from build123d import *

# Parameters (mm, degrees)
F0_R          = 38.3309835302
F0_R_2        = 24.0387523189
F1_DEPTH      = 101.6
F2_W          = 25.4
F2_H          = 50.8
F3_DEPTH      = 38.3319835302
F3_DEPTH_BACK = 38.3319835302
F4_R          = 4.4552500981
F5_DEPTH      = 25.4


with BuildPart() as f1:
    # F0 (on Top) → F1 (new body)
    with BuildSketch(Plane.XY):
        Circle(F0_R)
        Circle(F0_R_2, mode=Mode.SUBTRACT)
    extrude(amount=F1_DEPTH)

    # F2 (on Front) → F3 (cut, two sides)
    with BuildSketch(Plane.XZ) as f3_sk:
        with Locations((0, 50.8)):
            Rectangle(F2_W, F2_H)
    extrude(amount=-F3_DEPTH, mode=Mode.SUBTRACT)
    extrude(f3_sk.sketch, amount=F3_DEPTH_BACK, mode=Mode.SUBTRACT)

    # F4 (on face) → F5 (cut, through all)
    with BuildSketch(Plane.XY.offset(101.6)):
        with Locations((0, 31.9115035236)):
            Circle(F4_R)
    extrude(amount=-F5_DEPTH, mode=Mode.SUBTRACT)


solid = f1.part
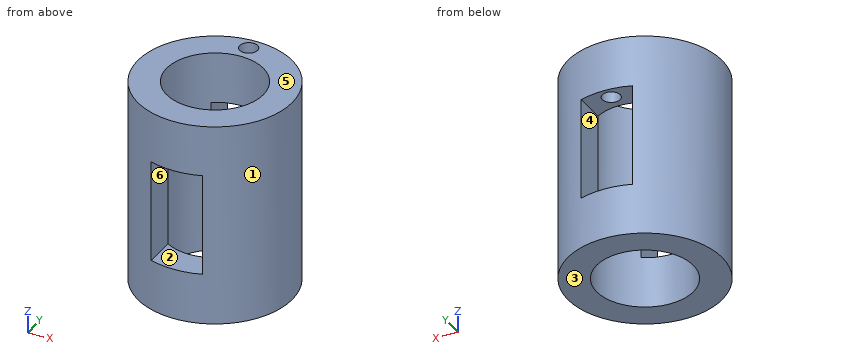
Could you check a few things on this model? Use its own coordinates, in mm. Face numbers are marked on the shaded views. A direction names the side the tool comes from. Give positions to 0.01 mm unless a question says otherwise; leave off trailing zeros. Loops run counter-clockwise (first coordinate to the right, second up) from the corner with the lowest first, then second, coordinate; pieces in that order, holes last. Notation, with made-up numbers: M -39.5,-6 L -35.5,-6 A14 cw -35.5,-1 Z; hole C 5,65.25 d9. An arc over 180 degrees is marked long. Answer as a JSON object with one key per item and string values.
Q1. For P1, Ø6, axis at y = 17, z = 21.5, coming from the +X side; P2, Ø6, axis at x = -27, z = 74, coming from the +Y side; P3, Ø4.5, axis at y = 31.5, z = 52.5, coming from the -X side, each with a flat end and sliding along its axis, tell me the tip position at first contact or that it passes through.
Values found:
{"P1": "stops at x = 35.68", "P2": "stops at y = 29.89", "P3": "stops at x = -24.77"}
Q2. If I drill on probe 1 along Y at (x, z) = (0, 80.5); probe 2 along X at (y, z) = (-0.5, 65.5); probe 3 along X at (y, z) = (-12, 79), over which ranges is the centre line in solid material (lowest first)? Write a range as [from, to].
Values found:
{"probe 1": "y = [-38.33, -24.04], [24.04, 27.46], [36.37, 38.33]", "probe 2": "x = [-38.33, -24.03], [24.03, 38.33]", "probe 3": "x = [-36.4, -20.83], [20.83, 36.4]"}
Q3. Suppose I cut it at D-D, the plane x = -9. List the corners of the cut face in (y, z) for me.
Values found:
{"outline": "M -37.26,0 L -22.29,0 L -22.29,25.4 L -37.26,25.4 Z; M -37.26,76.2 L -22.29,76.2 L -22.29,101.6 L -37.26,101.6 Z; M 22.29,0 L 37.26,0 L 37.26,25.4 L 22.29,25.4 Z; M 22.29,76.2 L 37.26,76.2 L 37.26,101.6 L 22.29,101.6 Z"}
Q4. If we mould it in two halves opening along X, with no side actions, what happens to the marked faces 1, 2, 3 and 4? For each: pulls with the +X half, pulls with the -X half, needs draft (parallel to the pull), parting line crosses it, or undercut.
Values found:
{"face 1": "parting line crosses it", "face 2": "undercut", "face 3": "needs draft", "face 4": "undercut"}
Q5. Suppose I cut it at C-C, the plane z = 53. List the corners of the cut face in (x, y) for me, plus the area to 3 significant figures.
Values found:
{"outline": "M -12.7,-36.17 L -12.7,-20.41 A24.04 cw -12.7,20.41 L -12.7,36.17 A38.33 ccw Z; M 12.7,-36.17 A38.33 ccw 12.7,36.17 L 12.7,20.41 A24.04 cw 12.7,-20.41 Z", "area": "2,050 mm²"}
Q6. For the marked faces 5 and 6, which set-ups out of +Z, -Z, +X, -X, +Y, -Y let a thin tool reach every point of the face, with its end or its side?
Values found:
{"face 5": "+Z, +X, -X, +Y, -Y", "face 6": "+Y, -Y"}
Q7. Suppose I cut it at B-B, the plane x = 0. List the corners of the cut face in (y, z) for me.
Values found:
{"outline": "M -38.33,0 L -24.04,0 L -24.04,25.4 L -38.33,25.4 Z; M -38.33,76.2 L -24.04,76.2 L -24.04,101.6 L -38.33,101.6 Z; M 24.04,0 L 38.33,0 L 38.33,25.4 L 24.04,25.4 Z; M 24.04,76.2 L 27.46,76.2 L 27.46,101.6 L 24.04,101.6 Z; M 36.37,76.2 L 38.33,76.2 L 38.33,101.6 L 36.37,101.6 Z"}
Q8. Suppose I cut it at A-A, the plane y = 0. List the corners of the cut face in (x, z) for me, plus the area to 3 significant figures.
Values found:
{"outline": "M -38.33,0 L -24.04,0 L -24.04,101.6 L -38.33,101.6 Z; M 24.04,0 L 38.33,0 L 38.33,101.6 L 24.04,101.6 Z", "area": "2,900 mm²"}
